The figure shows three views and two pictorial views of one solid part (mm, origin at its lowest corner). Answer the questions. A direction names the side the tool comes from. Give positions to 0.01 mm unless a question says otherwise; leave off trailing zeros. Loops run counter-clockwise (first coordinate to the right, second up) from the corner with the lowest first, then second, coordinate; pieces in that order, holes last. Notation, with made-up numbers: M -33.5,71.5 L -23.5,71.5 A14 ccw -23.5,96.5 Z; hole C 69,59 d1. An arc over 180 degrees is marked long. Write item = value, one per line. Start each with the question number.
1. The mould has two halves that part along Y. Classify the marked faces 5, 6 and 7: released by +Y, released by -Y, zero draft, split by the parting line, or undercut.
2. Section A-A on x = 40 is taken. Determine the outline of the cut face in (y, z).
3. Consider L1, parallel to Z at x = 71, y = 40; L2, parallel to Z at x = 69, y = 40; L3, parallel to X at y = 28.5, z = 62. Determine where each line is inside the solid, lowest interval first. Write a range as [from, to].
4. Flat-ended cylindrical pins translate along their axes: pin 1 Ø5.5 at (x, z) = (76.5, 38) entering from -Y; pin 2 Ø8 at (x, y) = (34.5, 20) entering from +Z; pin 3 Ø2 at (x, z) = (77, 39.5) entering from +Y; pin 4 Ø5.5 at (x, z) = (3, 37) entering from +Y. Find the tip coordinate at first contact, or state that the pin passes through.
5. Section C-C on y = 40 is taken. Give the number of separate pieces and of enclosed holes in the cut face, plus the area to 3 significant figures.
6. For the marked faces 1, 2, 3 and 4, determine the directions among +Z, -Z, +X, -X, +Y, -Y from which every point of the face is accessible in a straight line to the end or side of a thin tool.
7. Section B-B on z = 49 is taken. Determine the outline of the cut face in (x, y) (1 decimal).
8. Section D-D on x = 69 is taken. Determine the outline of the cut face in (y, z), plus the area to 3 significant figures.
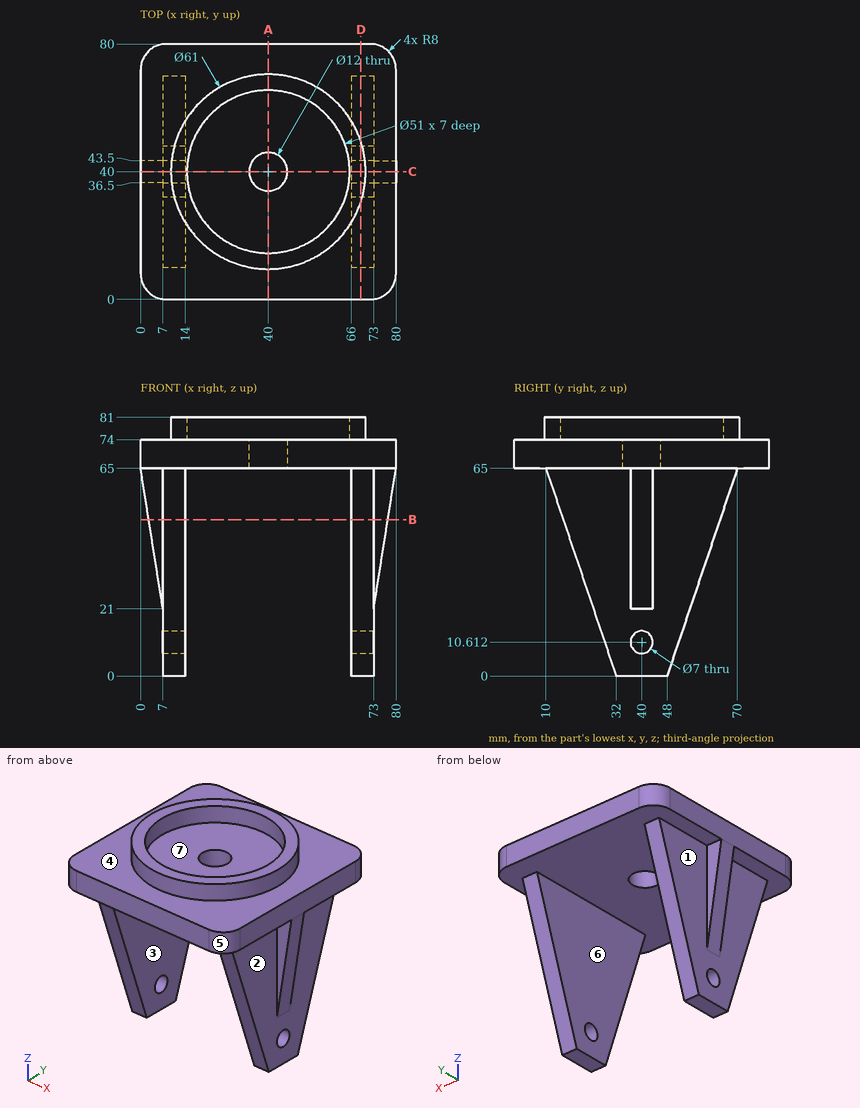
Verdict:
q1.face_5 = released by -Y
q1.face_6 = zero draft
q1.face_7 = undercut
q2.outline = M 0,65 L 34,65 L 34,74 L 14.5,74 L 14.5,81 L 9.5,81 L 9.5,74 L 0,74 Z; M 46,65 L 80,65 L 80,74 L 70.5,74 L 70.5,81 L 65.5,81 L 65.5,74 L 46,74 Z
q3.L1 = [0, 7.11], [14.11, 74]
q3.L2 = [0, 7.11], [14.11, 81]
q3.L3 = [7, 14], [66, 73]
q4.pin_1 = 36.5
q4.pin_2 = 74
q4.pin_3 = through
q4.pin_4 = 43.5
q5.separate_pieces = 4
q5.enclosed_holes = 0
q5.area = 1,800 mm2
q6.face_1 = -Z, -X
q6.face_2 = -Z, +X
q6.face_3 = -Z, +Y, -Y
q6.face_4 = +Z
q7.outline = M 2.5,36.5 L 7,36.5 L 7,15.4 L 14,15.4 L 14,64.6 L 7,64.6 L 7,43.5 L 2.5,43.5 Z; M 66,15.4 L 73,15.4 L 73,36.5 L 77.5,36.5 L 77.5,43.5 L 73,43.5 L 73,64.6 L 66,64.6 Z
q8.outline = M 0,65 L 10,65 L 32,0 L 48,0 L 70,65 L 80,65 L 80,74 L 49.45,74 L 49.45,81 L 30.55,81 L 30.55,74 L 0,74 Z; hole C 40,10.61 d7
q8.area = 3,280 mm2
